The figure shows three views and two pictorial views of one solid part (mm, origin at its lowest corner). Answer the questions. A direction names the side the tool comes from. Coordinates: 2 decimals unless noted, no trailing zeros. Loops run counter-clockwise (first coordinate to the right, second up) from the corner with the lowest first, then second, coordinate; pieces in that order, holes last. Notation, with made-up numbers: M 61,43.25 L 67,43.25 A14 ccw 67,69.25 Z; hole C 1.5,5 d5. An arc over 180 degrees is marked long. Return JSON: item names as keys, results as strings. Group by question number.
1. Section C-C (x = 2.5) is taken. Count the separate pieces of the cut face and the enclosed holes in it, then the cut area to 4 significant figures.
2. Straight lines are drawn through the part: L1, parallel to X at y = 0.85, z = 15.5; L2, parallel to Z at x = 2.5, y = 5.7; L3, parallel to Y at x = 15, z = 7.75. For each, find the intervals that lie inside material, in ascending order. Write a range as from..to.
3. Section D-D (y = 5) is taken. Write down the section's boundary in (x, z), then the cut area to 3 significant figures.
4. Section A-A (z = 4.75) is taken. Write down the section's boundary in (x, y).
5. Section B-B (y = 7) is taken. Write down the section's boundary in (x, z).
6. Which of the six approach directions +Z, -Z, +X, -X, +Y, -Y give full straight-line access (tool end or side, diameter ignored) to the marked faces 1, 2 and 3?
7. Given P1, Ø5.5, axis at x = 1.5, y = 11.5, coming from the +Z side; P2, Ø4, axis at y = 10.5, z = 5.5, coming from the +X side; P3, Ø5, axis at x = 13.5, z = 5.5, coming from the -Y side; P4, Ø3.5, axis at x = 2.5, z = 15.5, coming from the +Y side, each flat-ended and moving along its own axis, determine where each tip first touches the part or whether it passes through.
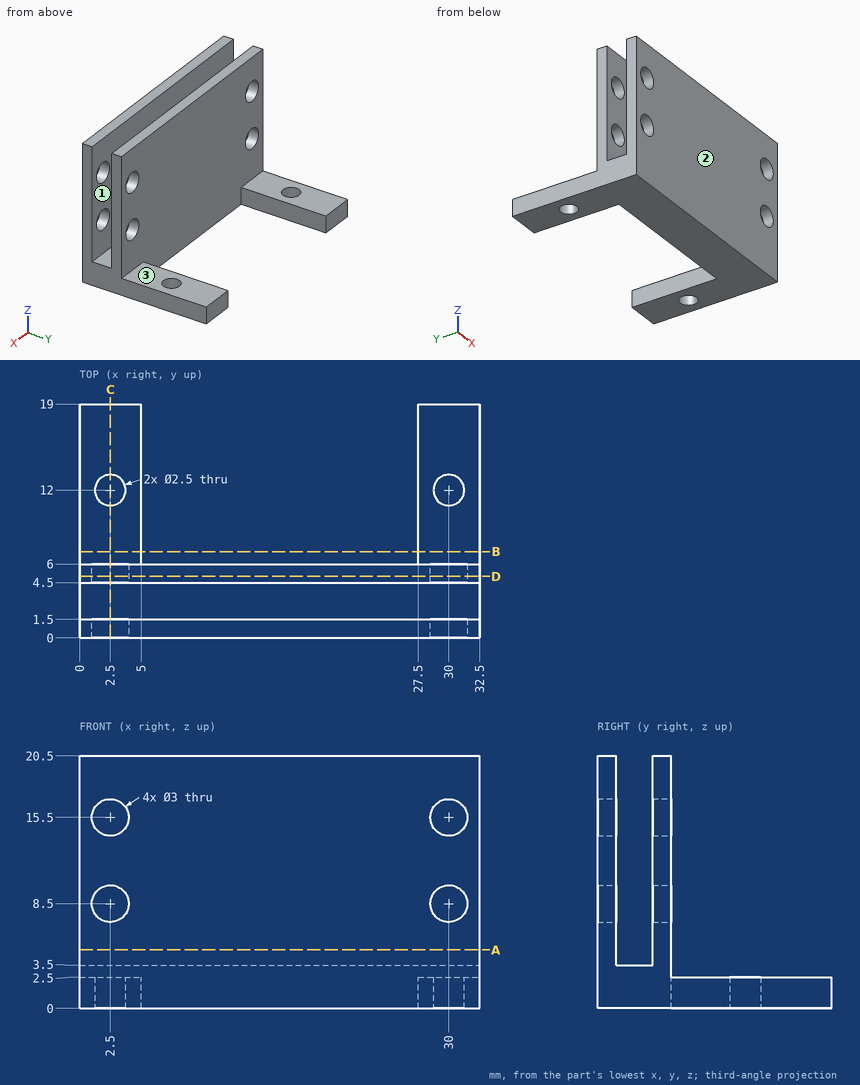
Worked out:
{
 "1": {"separate pieces": "6", "enclosed holes": "0", "area": "80.25 mm^2"},
 "2": {"L1": "0..1, 4..28.5, 31.5..32.5", "L2": "0..7, 10..14, 17..20.5", "L3": "0..1.5, 4.5..6"},
 "3": {"outline": "M 0,0 L 32.5,0 L 32.5,20.5 L 0,20.5 Z; hole C 2.5,8.5 d3; hole C 2.5,15.5 d3; hole C 30,8.5 d3; hole C 30,15.5 d3", "area": "638 mm^2"},
 "4": {"outline": "M 0,0 L 32.5,0 L 32.5,1.5 L 0,1.5 Z; M 0,4.5 L 32.5,4.5 L 32.5,6 L 0,6 Z"},
 "5": {"outline": "M 0,0 L 5,0 L 5,2.5 L 0,2.5 Z; M 27.5,0 L 32.5,0 L 32.5,2.5 L 27.5,2.5 Z"},
 "6": {"face 1": "+Z, +X, -X", "face 2": "+Z, -Z, +X, -X, -Y", "face 3": "+Z, +X, -X, +Y"},
 "7": {"P1": "z = 2.5", "P2": "through", "P3": "y = 0", "P4": "y = 6"}
}
